Check sheet for the modelled part. Datum: model origin and axes. Units: mm. A direction names the side the tool comes from. Coordinates: 2 decimals unless noted, no trailing zeros. Order: outer loops, then holes, each group sorted by start corner. A loop starts at its lowest first (then second) coordinate and runs counter-clockwise, first axis right, second up.
1. Draft check along Y on faces 1 (the flat face through (0, 4, -55)), 2 (the flat face through (100, 0, -38)), 3 (the cylindrical face through (193.67, 38.24, -73.07)). Enter one of: released by +Y, released by -Y, zero draft, split by the parting line, or undercut.
2. Cross-section at B-B (y = 38.1). Enter the section's corners in (x, z) (3 decimals).
3. Cross-section at D-D (x = 113.5). Enter the section's corners in (y, z), then the cut area to 3 significant figures.
4. Thickness scan on line 1 (X direction, y = 3, z = -25); line 2 (Y direction, x = 190.5, z = -75) (3 decimals); line 3 (X direction, y = 3.5, z = -25.4) (3 decimals). Record the ranges inside material, lowest first.
5. Cross-section at C-C (x = 12.7). Enter the section's corners in (y, z) (3 decimals), then the cut area to 3 significant figures.
6. Set-up check for faces 4 (the cylindrical face through (10.993, 40.777, -73.069)), 5 (the flat face through (100, 42, -69.85)): record each of +Z, -Z, +X, -X, +Y, -Y from which the full face is reachable in a straight line by a thin tool's end or side.
7. Gauge pin test, flat ends, axial feed: pin 1 Ø8.5 at (x, y) = (12.7, 19.05) entering from +Z; pin 2 Ø4 at (x, z) = (80.5, -11) entering from +Y; pin 3 Ø3 at (x, z) = (81.5, -41) entering from -Y. Record the tip position at first contact, or that the pin passes through.
8. Cross-section at A-A (z = -25.4). Enter the section's corners in (x, y) (3 decimals), then the cut area to 3 significant figures.
```python
from build123d import *

# Parameters (mm, degrees)
BOSS_EXTRUDE2_DEPTH = 203.2
SKETCH4_R           = 3.175
CUT_EXTRUDE1_DEPTH  = 71.628
SKETCH5_R           = 3.175
CUT_EXTRUDE2_DEPTH  = 244.602


with BuildPart() as part:
    # Sketch2 → Boss-Extrude2 (new body)
    with BuildSketch(Plane(origin=(0, 0, 0), x_dir=(0, 0, -1), z_dir=(1, 0, 0))):
        Polygon((0, 6.35), (0, 0), (76.2, 0), (76.2, 76.2), (69.85, 76.2), (69.85, 6.35), align=None)
    extrude(amount=BOSS_EXTRUDE2_DEPTH)

    # Sketch4 → Cut-Extrude1 (cut)
    with BuildSketch(Plane(origin=(0, 0, -76.2), x_dir=(-1, 0, 0), z_dir=(0, 0, -1))):
        with Locations((-190.5, 19.05)):
            Circle(SKETCH4_R)
        with Locations((-190.5, 38.1)):
            Circle(SKETCH4_R)
        with Locations((-12.7, 19.05)):
            Circle(SKETCH4_R)
        with Locations((-12.7, 38.1)):
            Circle(SKETCH4_R)
    extrude(amount=-CUT_EXTRUDE1_DEPTH, mode=Mode.SUBTRACT)

    # Sketch5 → Cut-Extrude2 (cut)
    with BuildSketch(Plane(origin=(0, 6.35, 0), x_dir=(1, 0, 0), z_dir=(0, 1, 0))):
        with Locations(Location((25.4, 25.4, 0), (0, 0, 270))):
            Circle(SKETCH5_R)
        with Locations(Location((177.8, 25.4, 0), (0, 0, 270))):
            Circle(SKETCH5_R)
        with Locations(Location((101.6, 25.4, 0), (0, 0, 270))):
            Circle(SKETCH5_R)
    extrude(amount=-CUT_EXTRUDE2_DEPTH, mode=Mode.SUBTRACT)


solid = part.part
```
Data:
1. face 1: zero draft
1. face 2: released by -Y
1. face 3: undercut
2. outline: (0, -76.2) - (9.525, -76.2) - (9.525, -69.85) - (0, -69.85) - close; (15.875, -76.2) - (187.325, -76.2) - (187.325, -69.85) - (15.875, -69.85) - close; (193.675, -76.2) - (203.2, -76.2) - (203.2, -69.85) - (193.675, -69.85) - close
3. outline: (0, -76.2) - (76.2, -76.2) - (76.2, -69.85) - (6.35, -69.85) - (6.35, 0) - (0, 0) - close
3. area: 927 mm2
4. line 1: x = 0 to 22.25, 28.55 to 98.45, 104.75 to 174.65, 180.95 to 203.2
4. line 2: y = 0 to 15.875, 22.225 to 34.925, 41.275 to 76.2
4. line 3: x = 0 to 22.225, 28.575 to 98.425, 104.775 to 174.625, 180.975 to 203.2
5. outline: (0, -76.2) - (15.875, -76.2) - (15.875, -69.85) - (6.35, -69.85) - (6.35, 0) - (0, 0) - close; (22.225, -76.2) - (34.925, -76.2) - (34.925, -69.85) - (22.225, -69.85) - close; (41.275, -76.2) - (76.2, -76.2) - (76.2, -69.85) - (41.275, -69.85) - close
5. area: 847 mm2
6. face 4: +Z, -Z
6. face 5: +Z, +X, -X, +Y
7. pin 1: stops at z = -69.85
7. pin 2: stops at y = 6.35
7. pin 3: stops at y = 0
8. outline: (0, 0) - (22.225, 0) - (22.225, 6.35) - (0, 6.35) - close; (28.575, 0) - (98.425, 0) - (98.425, 6.35) - (28.575, 6.35) - close; (104.775, 0) - (174.625, 0) - (174.625, 6.35) - (104.775, 6.35) - close; (180.975, 0) - (203.2, 0) - (203.2, 6.35) - (180.975, 6.35) - close
8. area: 1,170 mm2
